CAD build for the part. Positions are in the model's coordinates, mm. A direction names the side the tool comes from. Round coordinates to 2 decimals unless told otherwise and drop trailing zeros. Loops run counter-clockwise (first coordinate to the right, second up) from the corner with the lowest first, then second, coordinate; pieces in that order, holes last. Notation, with made-up numbers: (-25.5, 29) - (12.5, 29) arc R8 cw to (12.5, 37) - close; hole circle Ø9 at (26.5, 17). An arc over 180 degrees is marked (long way). One line per question, with ' | ' between items.
```python
from build123d import *

# Parameters (mm, degrees)
EXTRUDE1_DEPTH     = 85
SHELL1_T           = -1
SKETCH3_R          = 45
CUT_EXTRUDE1_DEPTH = 30


with BuildPart() as part:
    # Sketch1 → Extrude1 (new body)
    with BuildSketch(Plane(origin=(0, 0, 0), x_dir=(1, 0, 0), z_dir=(0, 1, 0))):
        Polygon((0, 30), (30, 0), (0, -30), (-30, 0), align=None)
    extrude(amount=EXTRUDE1_DEPTH)

    # Shell1
    shell1_openings = [part.faces().sort_by_distance(p)[0] for p in [
        (0, 85, 0),
        (0, 0, 0),
    ]]
    offset(amount=SHELL1_T, openings=shell1_openings, kind=Kind.INTERSECTION)

    # Sketch3 → Cut-Extrude1 (cut, symmetric)
    with BuildSketch(Plane(origin=(0, 0, 0), x_dir=(0, 0, -1), z_dir=(1, 0, 0))):
        with Locations((-30, 85)):
            Circle(SKETCH3_R)
    extrude(amount=CUT_EXTRUDE1_DEPTH, both=True, mode=Mode.SUBTRACT)


solid = part.part
```
(1) Probe L1, parallel to X at y = 45, z = -14; L2, parallel to X at y = 31.5, z = 21.5; L3, parallel to Z at x = -18, y = 26. List the from-to ranges inside material, lowest first.
Results found:
L1: x = -16 to -14.59, 14.59 to 16 | L2: x = -8.5 to -7.09, 7.09 to 8.5 | L3: z = -12 to -10.59, 10.59 to 12
(2) Cut at A-A, the plane y = 24. Write the cut outline in (x, z).
Results found:
outline: (-30, 0) - (0, -30) - (30, 0) - (0, 30) - close; hole (-28.59, 0) - (0, -28.59) - (28.59, 0) - (0, 28.59) - close
(3) Tool access for faces 1 (the face through (14.093, 32.461, -14.493)), 2 (the face through (16, 0, -13)): list every direction of +Z, -Z, +X, -X, +Y, -Y with a clear straight run to the whole face (end or side of a thin tool).
Results found:
face 1: +Y, -Y | face 2: +Z, -Z, +X, -X, -Y
(4) Cut at C-C, the plane z = -3.5. Write the cut outline in (x, y).
Results found:
outline: (-26.5, 0) - (-25.09, 0) - (-25.09, 54.95) - (-26.5, 54.95) - close; (25.09, 0) - (26.5, 0) - (26.5, 54.95) - (25.09, 54.95) - close
(5) Cut at B-B, the plane x = -17. Write the cut outline in (y, z), then the cut area to 3 significant figures.
Results found:
outline: (0, -13) - (71.73, -13) arc R45 cw to (67.81, -11.59) - (0, -11.59) - close; (0, 11.59) - (43.94, 11.59) arc R45 cw to (43.33, 13) - (0, 13) - close | area: 160 mm²
(6) Cut at D-D, the plane y = 42.5. Write the cut outline in (x, z).
Results found:
outline: (-30, 0) - (0, -30) - (30, 0) - (14.79, 15.21) - (13.38, 15.21) - (28.59, 0) - (0, -28.59) - (-28.59, 0) - (-13.38, 15.21) - (-14.79, 15.21) - close
(7) Drop flat-ended pins along their axis: P1, Ø4, axis at x = -13, y = 18, coming from the +Z side; P2, Ø4, axis at x = 17.5, y = 73, coming from the -Z side; P3, Ø5, axis at x = -20.5, z = -7.5, coming from the +Y side. Give the stop position or say it passes through.
Results found:
P1: stops at z = 19 | P2: stops at z = -14.5 | P3: stops at y = 64.3
